The listing builds one solid part. Answer for the finished solid, in the listing's coordinates (mm). Face numbers are marked on the shaded views. A direction names the side the tool comes from. Coordinates: 2 decimals unless noted, no trailing zeros. Order: outer loops, then holes, each group sorted by start corner. A loop starts at its lowest first (then second) coordinate and runs counter-clockwise, first axis right, second up.
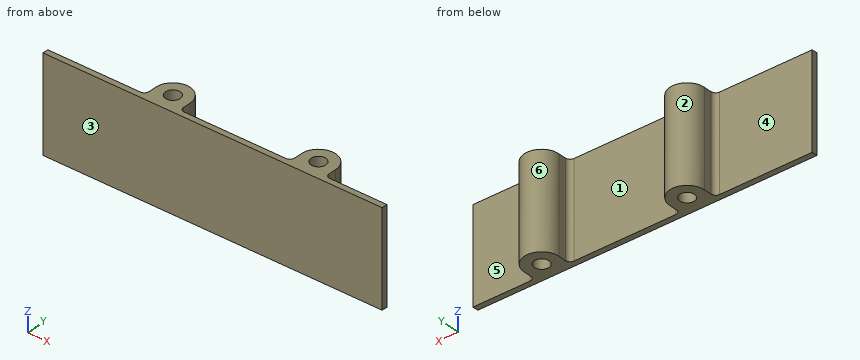
```python
from build123d import *

# Parameters (mm, degrees)
SKETCH1_W           = 399.27784
SKETCH1_H           = 3.175
BOSS_EXTRUDE1_DEPTH = 52.09999994
SKETCH3_R           = 4.075
BOSS_EXTRUDE2_DEPTH = 52.09999994
FILLET1_R           = 2.54
SKETCH5_W           = 212.27542
SKETCH5_H           = 58.123397562
CUT_EXTRUDE3_DEPTH  = 404.141539965


with BuildPart() as part:
    # Sketch1 → Boss-Extrude1 (new body)
    with BuildSketch(Plane.XY):
        with Locations((199.63892, 1.5875)):
            Rectangle(SKETCH1_W, SKETCH1_H)
    extrude(amount=BOSS_EXTRUDE1_DEPTH)

    # Sketch3 → Boss-Extrude2 (add)
    # profile 1 of 4: a face of its own
    with BuildSketch(Plane(origin=(0, 0, 0), x_dir=(-1, 0, 0), z_dir=(0, 0, -1))):
        with BuildLine():
            Line((-313.50704, 10.11428), (-313.50704, 3.175))
            Line((-313.50704, 3.175), (-303.97704, 3.175))
            Line((-303.97704, 3.175), (-294.44704, 3.175))
            Line((-294.44704, 3.175), (-294.44704, 10.11428))
            ThreePointArc((-294.44704, 10.11428), (-303.97704, 19.64428), (-313.50704, 10.11428))
        make_face()
        with Locations((-303.97704, 10.11428)):
            Circle(SKETCH3_R, mode=Mode.SUBTRACT)
    # profile 2 of 4: a face of its own
    with BuildSketch(Plane(origin=(0, 0, 0), x_dir=(-1, 0, 0), z_dir=(0, 0, -1))):
        with BuildLine():
            Line((-233.24304, 3.175), (-223.71304, 3.175))
            Line((-223.71304, 3.175), (-214.18304, 3.175))
            Line((-214.18304, 3.175), (-214.18304, 10.11428))
            ThreePointArc((-214.18304, 10.11428), (-223.71304, 19.64428), (-233.24304, 10.11428))
            Line((-233.24304, 10.11428), (-233.24304, 3.175))
        make_face()
        with Locations((-223.71304, 10.11428)):
            Circle(SKETCH3_R, mode=Mode.SUBTRACT)
    # profile 3 of 4: a face of its own
    with BuildSketch(Plane(origin=(0, 0, 0), x_dir=(-1, 0, 0), z_dir=(0, 0, -1))):
        with BuildLine():
            Line((-152.97904, 3.175), (-143.44904, 3.175))
            Line((-143.44904, 3.175), (-133.91904, 3.175))
            Line((-133.91904, 3.175), (-133.91904, 10.11428))
            ThreePointArc((-133.91904, 10.11428), (-143.44904, 19.64428), (-152.97904, 10.11428))
            Line((-152.97904, 10.11428), (-152.97904, 3.175))
        make_face()
        with Locations((-143.44904, 10.11428)):
            Circle(SKETCH3_R, mode=Mode.SUBTRACT)
    # profile 4 of 4: a face of its own
    with BuildSketch(Plane(origin=(0, 0, 0), x_dir=(-1, 0, 0), z_dir=(0, 0, -1))):
        with BuildLine():
            Line((-72.71504, 3.175), (-63.18504, 3.175))
            Line((-63.18504, 3.175), (-53.65504, 3.175))
            Line((-53.65504, 3.175), (-53.65504, 10.11428))
            ThreePointArc((-53.65504, 10.11428), (-63.18504, 19.64428), (-72.71504, 10.11428))
            Line((-72.71504, 10.11428), (-72.71504, 3.175))
        make_face()
        with Locations((-63.18504, 10.11428)):
            Circle(SKETCH3_R, mode=Mode.SUBTRACT)
    extrude(amount=-BOSS_EXTRUDE2_DEPTH)

    # Fillet1
    fillet1_edges = [part.edges().sort_by_distance(p)[0] for p in [
        (294.44704, 3.175, 26.04999997),
        (313.50704, 3.175, 26.04999997),
        (233.24304, 3.175, 26.04999997),
        (214.18304, 3.175, 26.04999997),
        (152.97904, 3.175, 26.04999997),
        (133.91904, 3.175, 26.04999997),
        (72.71504, 3.175, 26.04999997),
        (53.65504, 3.175, 26.04999997),
    ]]
    fillet(fillet1_edges, radius=FILLET1_R)

    # Sketch5 → Cut-Extrude3 (cut, through all)
    with BuildSketch(Plane(origin=(0, 0, 0), x_dir=(-1, 0, 0), z_dir=(0, 0, -1))):
        with Locations((-293.14013, 29.061698781)):
            Rectangle(SKETCH5_W, SKETCH5_H)
    extrude(amount=-CUT_EXTRUDE3_DEPTH, mode=Mode.SUBTRACT)


solid = part.part
```
1) Straight lines are drawn through the part: probe 1 along X at (y, z) = (9.75, 14); probe 2 along X at (y, z) = (13.5, 21); probe 3 along Y at (x, z) = (111.5, 29.5) (3 decimals). For each, find the intervals that lie inside material, in ascending order.
2) A cutting plane is placed at C-C, the plane y = 8. Write down the section's boundary in (x, z), plus the area to 3 significant figures.
3) For the marked faces 4, 5 and 6, determine the directions among +Z, -Z, +X, -X, +Y, -Y from which every point of the face is accessible in a straight line to the end or side of a thin tool.
4) Each of these flat-tipped pins is pushed along its axis until it touches: P1, Ø1.3, axis at y = 7, z = 18, coming from the +X side; P2, Ø15.5, axis at x = 17.5, z = 30.5, coming from the +Y side (3 decimals); P3, Ø7.5, axis at x = 143.45, y = 10.11, coming from the +Z side; P4, Ø5, axis at y = 7, z = 29.5, coming from the +X side. Where does it stop, or does it pass through?
5) A cutting plane is placed at B-B, the plane y = 18. Write down the section's boundary in (x, z).
6) A cutting plane is placed at A-A, the plane z = 48.5. Write down the section's boundary in (x, y) (3 decimals).
7) The mould has two halves that part along X. Classify the marked faces 1, 2 and 3: released by +X, released by -X, zero draft, split by the parting line, or undercut.
8) A cutting plane is placed at D-D, the plane x = 49. Write down the section's boundary in (y, z) (3 decimals), plus the area to 3 significant figures.
Working result:
1. probe 1: x = 53.66 to 59.13, 67.24 to 72.72, 133.92 to 139.39, 147.51 to 152.98
1. probe 2: x = 54.28 to 60.92, 65.45 to 72.09, 134.54 to 141.18, 145.72 to 152.36
1. probe 3: y = 0 to 3.175
2. outline: (53.66, 0) - (59.7, 0) - (59.7, 52.1) - (53.66, 52.1) - close; (66.67, 0) - (72.72, 0) - (72.72, 52.1) - (66.67, 52.1) - close; (133.92, 0) - (139.97, 0) - (139.97, 52.1) - (133.92, 52.1) - close; (146.93, 0) - (152.98, 0) - (152.98, 52.1) - (146.93, 52.1) - close
2. area: 1,260 mm2
3. face 4: +Z, -Z, -X, +Y
3. face 5: +Z, -Z, +X, +Y
3. face 6: +Z, -Z, +Y
4. P1: stops at x = 152.98
4. P2: stops at y = 3.175
4. P3: passes through
4. P4: stops at x = 153.29
5. outline: (57.83, 0) - (68.54, 0) - (68.54, 52.1) - (57.83, 52.1) - close; (138.1, 0) - (148.8, 0) - (148.8, 52.1) - (138.1, 52.1) - close
6. outline: (0, 0) - (187.002, 0) - (187.002, 3.175) - (155.519, 3.175) arc R2.54 cw to (152.979, 5.715) - (152.979, 10.114) arc R9.53 ccw to (133.919, 10.114) - (133.919, 5.715) arc R2.54 cw to (131.379, 3.175) - (75.255, 3.175) arc R2.54 cw to (72.715, 5.715) - (72.715, 10.114) arc R9.53 ccw to (53.655, 10.114) - (53.655, 5.715) arc R2.54 cw to (51.115, 3.175) - (0, 3.175) - close; hole circle Ø8.15 at (63.185, 10.114); hole circle Ø8.15 at (143.449, 10.114)
7. face 1: undercut
7. face 2: undercut
7. face 3: zero draft
8. outline: (0, 0) - (3.175, 0) - (3.175, 52.1) - (0, 52.1) - close
8. area: 165 mm2
